Geometry check sheet. Reference: drawing and pictorial views, mm from the part's lowest x, y, z. A direction names the side the tool comes from. Coordinates: 2 decimals unless noted, no trailing zeros. Loops run counter-clockwise (first coordinate to the right, second up) from the corner with the lowest first, then second, coordinate; pieces in that order, holes last. Notation, with made-up numbers: (27.25, 81.5) -> (69.25, 81.5) arc R16 cw to (69.25, 102.5) -> close; hole circle Ø11 at (52, 38.25). An arc over 180 degrees is marked (long way). Answer as a JSON object with one key per item and string values.
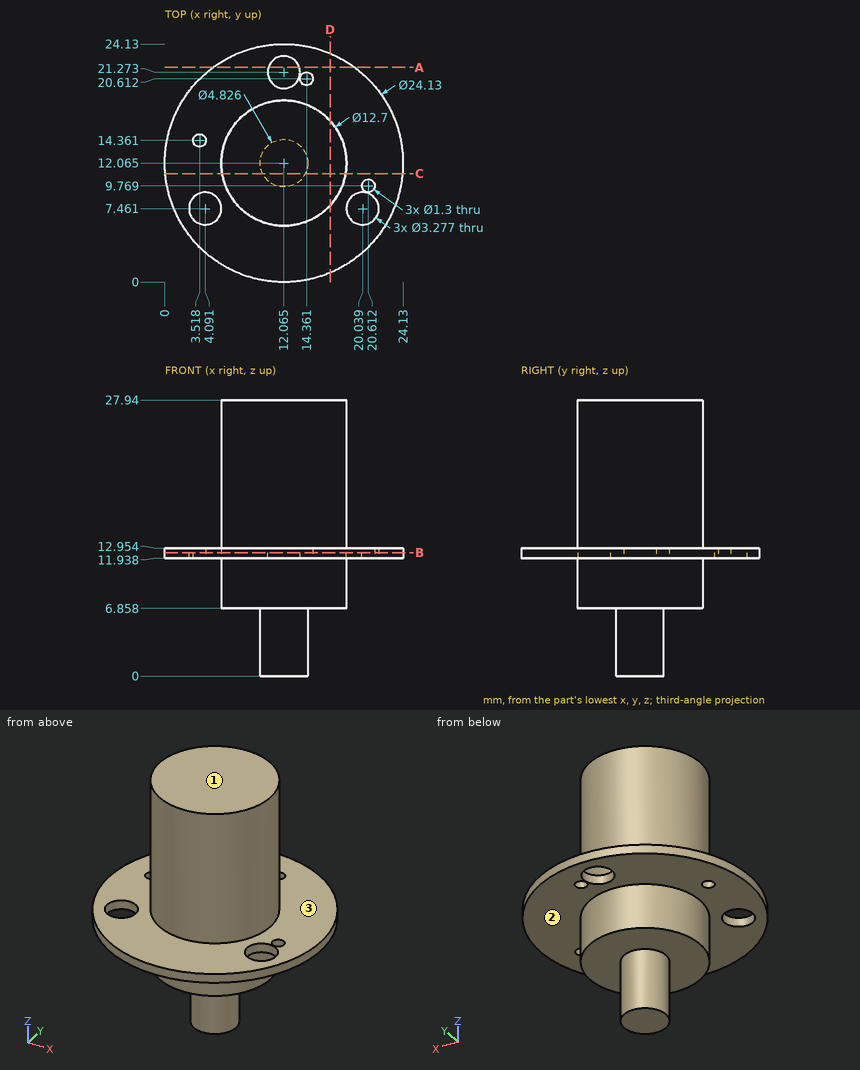
1. Section check D-D, the plane x = 16.75. Record the boundary of the cut face in (y, z) (1 decimal).
Evaluation:
{"outline": "(0.9, 11.9) -> (7.8, 11.9) -> (7.8, 6.9) -> (16.4, 6.9) -> (16.4, 11.9) -> (23.2, 11.9) -> (23.2, 13) -> (16.4, 13) -> (16.4, 27.9) -> (7.8, 27.9) -> (7.8, 13) -> (0.9, 13) -> close"}
2. Section check A-A, the plane y = 21.75. Record the boundary of the cut face in (x, z) (1 decimal).
Evaluation:
{"outline": "(4.9, 11.9) -> (10.5, 11.9) -> (10.5, 13) -> (4.9, 13) -> close; (13.6, 11.9) -> (19.3, 11.9) -> (19.3, 13) -> (13.6, 13) -> close"}
3. Tool access check on the marked faces 1, 2 and 3. Record the directions out of +Z, -Z, +X, -X, +Y, -Y that give a thin tool (end or side, any length) a straight path to the whole face; none if there is none.
Evaluation:
{"face 1": "+Z, +X, -X, +Y, -Y", "face 2": "-Z", "face 3": "+Z"}
4. Thickness scan on probe 1 along Z at (x, y) = (10.25, 5.75) (1 decimal); probe 2 along Z at (x, y) = (7.75, 14.75); probe 3 along Y at (x, z) = (7.75, 12.25). Record the ranges inside material, lowest first. Write a range as from..to.
Evaluation:
{"probe 1": "z = 11.9..13", "probe 2": "z = 6.86..27.94", "probe 3": "y = 0.8..23.33"}
5. Depth check by flat-ended pin: P1, Ø6, axis at x = 3.5, z = 24, coming from the +Y side (1 decimal); P2, Ø1, axis at x = 21, y = 20, coming from the -Z side; P3, Ø12, axis at x = 13, y = 10.5, coming from the -Z side; P4, Ø4.5, axis at x = 20.04, y = 7.46, coming from the +Z side. Enter the tip coordinate at first touch or a pass-through.
Evaluation:
{"P1": "stops at y = 15.1", "P2": "stops at z = 11.94", "P3": "stops at z = 0", "P4": "stops at z = 12.95"}
6. Section check C-C, the plane y = 11. Record the boundary of the cut face in (x, z) (1 decimal).
Evaluation:
{"outline": "(0, 11.9) -> (5.8, 11.9) -> (5.8, 6.9) -> (9.9, 6.9) -> (9.9, 0) -> (14.2, 0) -> (14.2, 6.9) -> (18.3, 6.9) -> (18.3, 11.9) -> (24.1, 11.9) -> (24.1, 13) -> (18.3, 13) -> (18.3, 27.9) -> (5.8, 27.9) -> (5.8, 13) -> (0, 13) -> close"}
7. Section check B-B, the plane z = 12.5. State how many separate pieces and enclosed holes the cut face has, then the cut area to 3 significant figures.
Evaluation:
{"separate pieces": "1", "enclosed holes": "6", "area": "428 mm^2"}
